Work out the finished part from the listing and answer in its coordinate system (mm). A direction names the side the tool comes from. Coordinates: 2 decimals unless noted, no trailing zeros. Order: outer loops, then holes, each group sorted by start corner. A loop starts at its lowest first (then second) coordinate and runs counter-clockwise, first axis right, second up.
1. A tool of negligible diameter and unlimited length cuts with its end or side. For faces 1 (the cylindrical face through (0.03, -17.93, -1.65)), 2 (the cylindrical face through (5.987, 0.246, 3.817)), 3 (the flat face through (0, -23, -2)), from which of +Z, -Z, +X, -X, +Y, -Y can it reach the whole face along a straight path? Write none if from no direction.
2. Find the intervals of material crossed by probe 1 along Y at (x, z) = (3, 6.75); probe 2 along Z at (x, y) = (0.25, -8.5); probe 3 along Y at (x, z) = (-2.25, -4.5), in increasing order.
3. The part is cut by section C-C, the plane y = -16.5. Give the vertices of the cut face in (x, z).
4. The part is cut by section B-B, the plane z = 0. Give the vertices of the cut face in (x, y).
5. The part is cut by section D-D, the plane y = -1.75. Give the vertices of the cut face in (x, z), then the cut area to 3 significant figures.
6. Flat-ended cylindrical pins translate along their axes: pin 1 Ø10 at (x, y) = (5, -2.5) entering from +Z; pin 2 Ø6 at (y, z) = (-5.5, -4) entering from +X; pin 3 Ø2 at (x, y) = (-5, -3.5) entering from +Z; pin 4 Ø4 at (y, z) = (-18.5, 4.5) entering from +X. Find the tip coordinate at first contact, or state that the pin passes through.
7. The part is cut by section A-A, the plane x = 0. Give the vertices of the cut face in (y, z).
```python
from build123d import *

# Parameters (mm, degrees)
SKETCH_1_R      = 7.1
EXTRUDE_1_DEPTH = 2
FILLET_1_R      = 1.5
SKETCH_2_R      = 6.4
EXTRUDE_2_DEPTH = 2
SKETCH_3_R      = 6
EXTRUDE_3_DEPTH = 13
SKETCH_4_R      = 0.75
EXTRUDE_4_DEPTH = 10
SKETCH_5_R      = 9.5
SKETCH_5_R_2    = 6
EXTRUDE_5_DEPTH = 3


with BuildPart() as part:
    # 草图1 → 拉伸1 (new body)
    with BuildSketch(Plane(origin=(0, 0, 0), x_dir=(1, 0, 0), z_dir=(0, 1, 0))):
        with Locations(Location((0, 0, 0), (0, 0, 270))):
            Circle(SKETCH_1_R)
    extrude(amount=EXTRUDE_1_DEPTH)

    # 圆角1
    fillet_1_edges = [part.edges().sort_by_distance(p)[0] for p in [
        (0, 2, -7.1),
    ]]
    fillet(fillet_1_edges, radius=FILLET_1_R)

    # 草图2 → 拉伸2 (add)
    with BuildSketch(Plane(origin=(0, 2, 0), x_dir=(-1, 0, 0), z_dir=(0, 1, 0))):
        with Locations(Location((0, 0, 0), (0, 0, 90))):
            Circle(SKETCH_2_R)
    extrude(amount=EXTRUDE_2_DEPTH)

    # 草图3 → 拉伸3 (add)
    with BuildSketch(Plane.XZ):
        with Locations(Location((0, 0, 0), (0, 0, 90))):
            Circle(SKETCH_3_R)
    extrude(amount=EXTRUDE_3_DEPTH)

    # 草图4 → 拉伸4 (add)
    with BuildSketch(Plane.XZ.offset(13)):
        with Locations(Location((0, -2.4, 0), (0, 0, 270))):
            Circle(SKETCH_4_R)
        with Locations(Location((0, 2.4, 0), (0, 0, 270))):
            Circle(SKETCH_4_R)
    extrude(amount=EXTRUDE_4_DEPTH)

    # 草图5 → 拉伸5 (add)
    with BuildSketch(Plane.XZ):
        with Locations(Location((0, 0, 0), (0, 0, 270))):
            Circle(SKETCH_5_R)
        with Locations(Location((0, 0, 0), (0, 0, 90))):
            Circle(SKETCH_5_R_2, mode=Mode.SUBTRACT)
    extrude(amount=EXTRUDE_5_DEPTH)


solid = part.part
```
Geometry says:
1. face 1: -Y
1. face 2: +Y
1. face 3: +Z, -Z, +X, -X, -Y
2. probe 1: y = -3 to 0
2. probe 2: z = -5.99 to 5.99
2. probe 3: y = -13 to 4
3. outline: circle Ø1.5 at (0, -2.4); circle Ø1.5 at (0, 2.4)
4. outline: (-9.5, -3) - (-6, -3) - (-6, -13) - (6, -13) - (6, -3) - (9.5, -3) - (9.5, 0) - (7.1, 0) - (7.1, 0.5) arc R1.5 ccw to (5.6, 2) - (6.4, 2) - (6.4, 4) - (-6.4, 4) - (-6.4, 2) - (-5.6, 2) arc R1.5 ccw to (-7.1, 0.5) - (-7.1, 0) - (-9.5, 0) - close
5. outline: circle Ø19 at (0, 0)
5. area: 284 mm2
6. pin 1: stops at z = 9.5
6. pin 2: stops at x = 9.21
6. pin 3: stops at z = 8.55
6. pin 4: stops at x = 0.74
7. outline: (-23, -3.15) - (-13, -3.15) - (-13, -6) - (-3, -6) - (-3, -9.5) - (0, -9.5) - (0, -7.1) - (0.5, -7.1) arc R1.5 ccw to (2, -5.6) - (2, -6.4) - (4, -6.4) - (4, 6.4) - (2, 6.4) - (2, 5.6) arc R1.5 ccw to (0.5, 7.1) - (0, 7.1) - (0, 9.5) - (-3, 9.5) - (-3, 6) - (-13, 6) - (-13, 3.15) - (-23, 3.15) - (-23, 1.65) - (-13, 1.65) - (-13, -1.65) - (-23, -1.65) - close
